Input: part model. Units: mm. Frame: model coordinates. Coordinates: 2 decimals unless noted, no trailing zeros. Order: outer loops, then holes, each group sorted by start corner. A loop starts at its lowest first (then second) coordinate and runs counter-clockwise, first axis right, second up. Notation, with made-up numbers: (67, -32) -> (84, -32) arc R7 cw to (84, -24) -> close; hole circle Ø4 at (82.5, 13.25). An arc over 180 degrees is marked (long way). Use one line per item in the form item = value. Start each with the question number.
1) Ray query, line 1 along Z through (x, y) = (6.75, 243.5); line 2 along X through (y, z) = (423.5, 8.5); line 3 along Z through (x, y) = (9.7, -50). Return the intervals inside material, ascending.
2) Section query B-B on y = 375. Output: boundary loops of the cut face in (x, z), then the cut area to 3 significant figures.
3) Pin query (flat end, axial travel): pin 1 (14.5 mm diameter, centred on y = -50, z = 0, fed in from +X). Return the tip coordinate at first contact, or that it passes through.
4) Section query A-A on x = -1.25. Output: boundary loops of the cut face in (y, z).
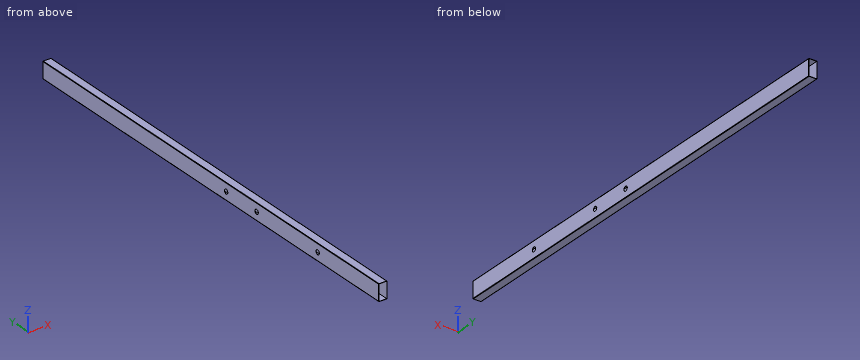
from build123d import *

# Parameters (mm, degrees)
F0_W     = 19
F0_H     = 39
F1_DEPTH = 550
F3_D     = 11
F3_DEPTH = 30
F3_TIP   = 3.3047334047


# Not quite as in the source:
# - a feature names something its author has since deleted; it is built from what else it names


with BuildPart() as f1:
    # F0 (on Front) → F1 (new body, symmetric)
    with BuildSketch(Plane.XZ):
        with BuildLine():
            Line((9, 20), (-9, 20))
            ThreePointArc((-9, 20), (-9.7071067812, 19.7071067812), (-10, 19))
            Line((-10, 19), (-10, -19))
            ThreePointArc((-10, -19), (-9.7071067812, -19.7071067812), (-9, -20))
            Line((-9, -20), (9, -20))
            ThreePointArc((9, -20), (9.7071067812, -19.7071067812), (10, -19))
            Line((10, -19), (10, 19))
            ThreePointArc((10, 19), (9.7071067812, 19.7071067812), (9, 20))
        make_face()
        Rectangle(F0_W, F0_H, mode=Mode.SUBTRACT)
    extrude(amount=F1_DEPTH, both=True)

    # F3
    with Locations(Plane.YZ.offset(10)):
        with Locations((-50, 0), (-150, 0), (-350, 0)):
            Hole(F3_D / 2, depth=F3_DEPTH)
            with Locations((0, 0, -(F3_DEPTH + F3_TIP / 2))):  # 118° drill point
                Cone(0, F3_D / 2, F3_TIP, mode=Mode.SUBTRACT)


solid = f1.part
Answers below:
q1.line_1 = -20 to -19.5, 19.5 to 20
q1.line_2 = -10 to -9.5, 9.5 to 10
q1.line_3 = -19.71 to -5.5, 5.5 to 19.71
q2.outline = (-10, -19) arc R1 ccw to (-9, -20) -> (9, -20) arc R1 ccw to (10, -19) -> (10, 19) arc R1 ccw to (9, 20) -> (-9, 20) arc R1 ccw to (-10, 19) -> close; hole (-9.5, -19.5) -> (9.5, -19.5) -> (9.5, 19.5) -> (-9.5, 19.5) -> close
q2.area = 58.1 mm^2
q3.pin_1 = 10
q4.outline = (-550, -20) -> (550, -20) -> (550, -19.5) -> (-550, -19.5) -> close; (-550, 19.5) -> (550, 19.5) -> (550, 20) -> (-550, 20) -> close
